Source: CAD feature listing. Evaluate the final solid. Frame: model axes, mm. Give positions to 0.01 mm unless a question says otherwise; leave off trailing zeros. Order: outer loops, then holes, each group sorted by start corner. A loop starts at its lowest first (then second) coordinate and runs counter-clockwise, first axis right, second up. Notation, with made-up numbers: (41.25, 5) -> (85.25, 5) arc R20 ccw to (85.25, 29) -> close; hole circle Ø7 at (54, -23.75). An arc over 180 degrees is marked (long way). Answer in a Markdown table with one row per item.
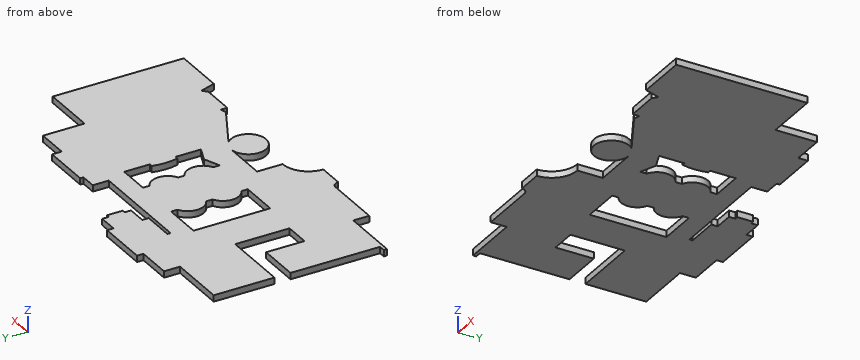
```python
from build123d import *

# Parameters (mm, degrees)
F1_DEPTH = 3.175


# Not quite as in the source:
# - ends of sketch curves that miss each other by under 0.0002 mm in the source are joined


with BuildPart() as f1:
    # F0 (on Top) → F1 (new body)
    with BuildSketch(Plane.XY):
        with BuildLine():
            Line((-34.925, 35.7325066477), (-55.5625, 35.7325066477))
            Line((-55.5625, 35.7325066477), (-55.5625, -8.7174933523))
            Line((-55.5625, -8.7174933523), (-58.7375, -8.7174933523))
            Line((-58.7375, -8.7174933523), (-58.7375, -10.3049933523))
            Line((-58.7375, -10.3049933523), (-30.1625, -10.3049933523))
            Line((-30.1625, -10.3049933523), (-30.1625, -18.2424933523))
            Line((-30.1625, -18.2424933523), (-1.5875, -18.2424933523))
            ThreePointArc((-1.5875, -18.2424933523), (0.6575640303, -19.172429322), (1.5875, -21.4174933523))
            Line((1.5875, -21.4174933523), (14.2875, -21.4174933523))
            ThreePointArc((14.2875, -21.4174933523), (18.0072438789, -12.4372372312), (26.9875, -8.7174933523))
            Line((26.9875, -8.7174933523), (26.9875, 3.9825066477))
            Line((26.9875, 3.9825066477), (49.2125, 3.9825066477))
            ThreePointArc((49.2125, 3.9825066477), (52.3581189283, 3.3961819464), (55.0812659129, 1.7159541056))
            Line((55.0812659129, 1.7159541056), (77.7875, -10.3049933523))
            Line((77.7875, -10.3049933523), (80.8780316716, -9.5775052173))
            Line((80.8780316716, -9.5775052173), (80.8780316716, -12.7525052173))
            Line((80.8780316716, -12.7525052173), (96.7530316716, -12.7525052173))
            Line((96.7530316716, -12.7525052173), (99.1648957133, -10.6876718476))
            Line((99.1648957133, -10.6876718476), (101.6, -18.2424933523))
            Line((101.6, -18.2424933523), (104.775, -18.2424933523))
            Line((104.775, -18.2424933523), (119.0625, -18.2424933523))
            Line((119.0625, -18.2424933523), (127, -18.2424933523))
            Line((127, -18.2424933523), (127, 46.8450066477))
            Line((127, 46.8450066477), (100.0125, 46.8450066477))
            Line((100.0125, 46.8450066477), (100.0125, 67.4825066477))
            Line((100.0125, 67.4825066477), (84.1375, 67.4825066477))
            Line((84.1375, 67.4825066477), (84.1375, 72.2450066477))
            Line((84.1375, 72.2450066477), (66.675, 72.2450066477))
            Line((66.675, 72.2450066477), (60.325, 72.2450066477))
            Line((60.325, 72.2450066477), (60.325, 70.6575066477))
            Line((60.325, 70.6575066477), (52.3875, 70.6575066477))
            Line((52.3875, 70.6575066477), (52.3875, 62.7200066477))
            Line((52.3875, 62.7200066477), (0, 62.7200066477))
            Line((0, 62.7200066477), (0, 64.3075066477))
            Line((0, 64.3075066477), (15.875, 64.3075066477))
            Line((15.875, 64.3075066477), (15.875, 67.4825066477))
            Line((15.875, 67.4825066477), (25.4, 67.4825066477))
            Line((25.4, 67.4825066477), (25.4, 70.6575066477))
            Line((25.4, 70.6575066477), (26.9875, 70.6575066477))
            Line((26.9875, 70.6575066477), (26.9875, 78.5950066477))
            Line((26.9875, 78.5950066477), (25.4, 78.5950066477))
            Line((25.4, 78.5950066477), (25.4, 81.7700066477))
            Line((25.4, 81.7700066477), (15.875, 81.7700066477))
            Line((15.875, 81.7700066477), (15.875, 84.9450066477))
            Line((15.875, 84.9450066477), (-9.525, 84.9450066477))
            Line((-9.525, 84.9450066477), (-9.525, 81.7700066477))
            Line((-9.525, 81.7700066477), (-26.9875, 81.7700066477))
            Line((-26.9875, 81.7700066477), (-26.9875, 73.8325066477))
            Line((-26.9875, 73.8325066477), (-55.5625, 73.8325066477))
            Line((-55.5625, 73.8325066477), (-55.5625, 43.6700066477))
            Line((-55.5625, 43.6700066477), (-22.225, 43.6700066477))
            Line((-22.225, 43.6700066477), (-22.225, 16.6825066477))
            Line((-22.225, 16.6825066477), (-34.925, 16.6825066477))
            Line((-34.925, 16.6825066477), (-34.925, 35.7325066477))
        make_face()
        Polygon((-3.175, 53.1950066477), (15.875, 53.1950066477), (15.875, 50.0200066477), (15.875, 35.7325066477), (15.875, 32.5575066477), (15.875, 18.2700066477), (15.875, 15.0950066477), (-3.175, 15.0950066477), align=None, mode=Mode.SUBTRACT)
        Polygon((39.6875, 50.0200066477), (39.6875, 53.1950066477), (55.5625, 53.1950066477), (55.5625, 40.4950066477), (55.5625, 27.7950066477), (55.5625, 15.0950066477), (47.625, 18.2700066477), (39.6875, 15.0950066477), (39.6875, 18.2700066477), (39.6875, 32.5575066477), (39.6875, 35.7325066477), align=None, mode=Mode.SUBTRACT)
        with BuildLine():
            Line((15.875, 35.7325066477), (15.875, 50.0200066477))
            ThreePointArc((15.875, 50.0200066477), (11.4771704008, 42.8762566477), (15.875, 35.7325066477))
        make_face()
        with BuildLine():
            Line((15.875, 18.2700066477), (15.875, 32.5575066477))
            ThreePointArc((15.875, 32.5575066477), (11.4771704008, 25.4137566477), (15.875, 18.2700066477))
        make_face()
        with BuildLine():
            ThreePointArc((39.6875, 35.7325066477), (44.0853295992, 42.8762566477), (39.6875, 50.0200066477))
            Line((39.6875, 50.0200066477), (39.6875, 35.7325066477))
        make_face()
        with BuildLine():
            ThreePointArc((39.6875, 18.2700066477), (44.0853295992, 25.4137566477), (39.6875, 32.5575066477))
            Line((39.6875, 32.5575066477), (39.6875, 18.2700066477))
        make_face()
        with BuildLine():
            Line((55.5625, 27.7950066477), (55.5625, 40.4950066477))
            Line((55.5625, 40.4950066477), (53.975, 40.4950066477))
            ThreePointArc((53.975, 40.4950066477), (53.1818915421, 34.1450066477), (53.975, 27.7950066477))
            Line((53.975, 27.7950066477), (55.5625, 27.7950066477))
        make_face()
        with BuildLine():
            ThreePointArc((55.0812659129, 1.7159541056), (52.3581189283, 3.3961819464), (49.2125, 3.9825066477))
            Line((49.2125, 3.9825066477), (49.2125, -13.4799933523))
            ThreePointArc((49.2125, -13.4799933523), (55.3864260832, -10.9226694355), (57.94375, -4.7487433523))
            ThreePointArc((57.94375, -4.7487433523), (57.1961203861, -1.2136999165), (55.0812659129, 1.7159541056))
        make_face()
        with BuildLine():
            Line((49.2125, -13.4799933523), (49.2125, 3.9825066477))
            ThreePointArc((49.2125, 3.9825066477), (40.48125, -4.7487433523), (49.2125, -13.4799933523))
        make_face()
    extrude(amount=F1_DEPTH)


solid = f1.part
```
(1) Ray query, probe 1 along Y at (x, z) = (5, 2.75) (1 decimal); probe 2 along Y at (x, z) = (-30.5, 1.1) (1 decimal); probe 3 along Y at (x, z) = (-35, 0.7) (1 decimal). Return the intervals inside material, ascending.
A:
| item | result |
|---|---|
| probe 1 | y = -21.4 to 15.1, 53.2 to 62.7, 64.3 to 84.9 |
| probe 2 | y = -10.3 to 16.7, 43.7 to 73.8 |
| probe 3 | y = -10.3 to 35.7, 43.7 to 73.8 |
(2) First-contact query: pin 1 Ø1 at (x, z) = (-29.5, 2) entering from +Y; pin 2 Ø1 at (x, z) = (88, 1) entering from +Y; pin 3 Ø1 at (y, z) = (66, 1) entering from +X. Flat tips, straight axial feed; report the tip coordinate or a pass-through.
A:
| item | result |
|---|---|
| pin 1 | stops at y = 73.83 |
| pin 2 | stops at y = 67.48 |
| pin 3 | stops at x = 100.01 |
(3) Section query B-B (y = 6.5). Return the cut outline in (x, z) (1 decimal).
A:
| item | result |
|---|---|
| outline | (-55.6, 0) -> (127, 0) -> (127, 3.2) -> (-55.6, 3.2) -> close |
(4) Section query A-A (z = 1.9). Give the number of separate pieces and of enclosed holes in the cut face, plus the area to 3 significant figures.
A:
| item | result |
|---|---|
| separate pieces | 1 |
| enclosed holes | 2 |
| area | 13,400 mm^2 |
(5) Section query C-C (x = 109). Return the cut outline in (y, z) (1 decimal), plus the area to 3 significant figures.
A:
| item | result |
|---|---|
| outline | (-18.2, 0) -> (46.8, 0) -> (46.8, 3.2) -> (-18.2, 3.2) -> close |
| area | 207 mm^2 |
